```python
from build123d import *

# Parameters (mm, degrees)
SKETCH1_R           = 25
BOSS_EXTRUDE1_DEPTH = 21
SKETCH2_R           = 28
BOSS_EXTRUDE2_DEPTH = 1
SKETCH3_R           = 28
BOSS_EXTRUDE3_DEPTH = 1
SKETCH4_R           = 15
BOSS_EXTRUDE4_DEPTH = 15
SKETCH5_R           = 4
BOSS_EXTRUDE5_DEPTH = 30
SKETCH6_R           = 4
BOSS_EXTRUDE6_DEPTH = 30


with BuildPart() as part:
    # Sketch1 → Boss-Extrude1 (new body)
    with BuildSketch(Plane(origin=(0, 0, 0), x_dir=(1, 0, 0), z_dir=(0, 1, 0))):
        Circle(SKETCH1_R)
    extrude(amount=BOSS_EXTRUDE1_DEPTH)

    # Sketch2 → Boss-Extrude2 (add)
    with BuildSketch(Plane(origin=(0, 0, 0), x_dir=(1, 0, 0), z_dir=(0, 1, 0))):
        Circle(SKETCH2_R)
    extrude(amount=BOSS_EXTRUDE2_DEPTH)

    # Sketch3 → Boss-Extrude3 (add)
    with BuildSketch(Plane(origin=(0, 21, 0), x_dir=(1, 0, 0), z_dir=(0, 1, 0))):
        Circle(SKETCH3_R)
    extrude(amount=BOSS_EXTRUDE3_DEPTH)

    # Sketch4 → Boss-Extrude4 (add)
    with BuildSketch(Plane(origin=(0, 22, 0), x_dir=(1, 0, 0), z_dir=(0, 1, 0))):
        Circle(SKETCH4_R)
    extrude(amount=BOSS_EXTRUDE4_DEPTH)

    # Sketch5 → Boss-Extrude5 (add)
    with BuildSketch(Plane(origin=(0, 37, 0), x_dir=(1, 0, 0), z_dir=(0, 1, 0))):
        Circle(SKETCH5_R)
    extrude(amount=BOSS_EXTRUDE5_DEPTH)

    # Sketch6 → Boss-Extrude6 (add)
    with BuildSketch(Plane(origin=(0, 0, 0), x_dir=(1, 0, 0), z_dir=(0, 1, 0))):
        Circle(SKETCH6_R)
    extrude(amount=-BOSS_EXTRUDE6_DEPTH)


solid = part.part
```
Model file for the job. Use its own axes, mm. A direction names the side the tool comes from. Give positions to 0.01 mm unless a question says otherwise; leave off trailing zeros. Loops run counter-clockwise (first coordinate to the right, second up) from the corner with the lowest first, then second, coordinate; pieces in that order, holes last. Notation, with made-up numbers: (39.5, 31) - (91.5, 31) arc R20 cw to (91.5, 61) - close; hole circle Ø10 at (39.5, 39). An arc over 180 degrees is marked (long way). One line per item, written item: value. Start each with the question number.
1. Slice it at A-A (x = 0). List the corners of the cut face in (y, z), plus the area to 3 significant figures.
2. Pin check, flat tips, straight feed: pin 1 (8 mm diameter, centred on x = -15.5, z = -15, fed in from +Y); pin 2 (1.5 mm diameter, centred on y = 14, z = 11, fed in from -X); pin 3 (2 mm diameter, centred on y = 12.5, z = 10.5, fed in from +X); pin 4 (17 mm diameter, centred on x = -1.5, z = -9.5, fed in from +Y). Stop position of each tip, or through.
3. Slice it at D-D (z = 13.5). List the corners of the cut face in (x, y), plus the area to 3 significant figures.
4. Probe L1, parallel to Y at x = -7, z = 19; L2, parallel to Y at x = 5.5, z = 11; L3, parallel to Z at x = -0.5, y = 26.5. List the from-to ranges inside material, lowest first. Write a range as from..to.
5. Slice it at B-B (z = 0). List the corners of the cut face in (x, y).
6. Slice it at C-C (y = 40). List the corners of the cut face in (x, z), plus the area to 3 significant figures.
7. Which spindle directions (+Z, -Z, +X, -X, +Y, -Y) get a long thin tool onto all of the face, cutting with end or side? Do faces 1 (the flat face through (-11, 1, -23)), 2 (the flat face through (3, 37, 3)), 3 (the cylindrical face through (25.865, 21.493, 10.724)), 4 (the cylindrical face through (-0.867, -14.79, 3.905)). Say none if no direction does.
8. Pull direction Y, two halves, no side cores. Call faces 5 (the flat face through (0, 67, 0)), 6 (the flat face through (0, -30, 0)), 7 (the cylindrical face through (25.865, 0.493, 10.724)), 8 (the cylindrical face through (23.846, 10.86, -7.509)): pulls with the +Y half, pulls with the -Y half, needs draft (parallel to the pull), parting line crosses it, or undercut.
Solution:
1. outline: (-30, -4) - (0, -4) - (0, -28) - (1, -28) - (1, -25) - (21, -25) - (21, -28) - (22, -28) - (22, -15) - (37, -15) - (37, -4) - (67, -4) - (67, 4) - (37, 4) - (37, 15) - (22, 15) - (22, 28) - (21, 28) - (21, 25) - (1, 25) - (1, 28) - (0, 28) - (0, 4) - (-30, 4) - close
1. area: 2,040 mm^2
2. pin 1: stops at y = 22
2. pin 2: stops at x = -22.8
2. pin 3: stops at x = 23.12
2. pin 4: stops at y = 67
3. outline: (-24.53, 0) - (24.53, 0) - (24.53, 1) - (21.04, 1) - (21.04, 21) - (24.53, 21) - (24.53, 22) - (6.54, 22) - (6.54, 37) - (-6.54, 37) - (-6.54, 22) - (-24.53, 22) - (-24.53, 21) - (-21.04, 21) - (-21.04, 1) - (-24.53, 1) - close
3. area: 1,140 mm^2
4. L1: y = 0..22
4. L2: y = 0..37
4. L3: z = -14.99..14.99
5. outline: (-28, 0) - (-4, 0) - (-4, -30) - (4, -30) - (4, 0) - (28, 0) - (28, 1) - (25, 1) - (25, 21) - (28, 21) - (28, 22) - (15, 22) - (15, 37) - (4, 37) - (4, 67) - (-4, 67) - (-4, 37) - (-15, 37) - (-15, 22) - (-28, 22) - (-28, 21) - (-25, 21) - (-25, 1) - (-28, 1) - close
6. outline: circle Ø8 at (0, 0)
6. area: 50.3 mm^2
7. face 1: none
7. face 2: +Y
7. face 3: +Y, -Y
7. face 4: -Y
8. face 5: pulls with the +Y half
8. face 6: pulls with the -Y half
8. face 7: needs draft
8. face 8: undercut
